Check sheet for the modelled part. Datum: model origin and axes. Units: mm. Face numbers are marked on the shaded views. Give positions to 0.01 mm unless a question says otherwise; leave off trailing zeros. Loops run counter-clockwise (first coordinate to the right, second up) from the corner with the lowest first, then second, coordinate; pieces in that order, holes last. Notation, with made-up numbers: (-34, 86.5) - (11, 86.5) arc R10 cw to (11, 97.5) - close; hole circle Ø7 at (67, 52). An arc over 180 degrees is marked (long way). Use CSV: the item, a comma, the result in double quotes.
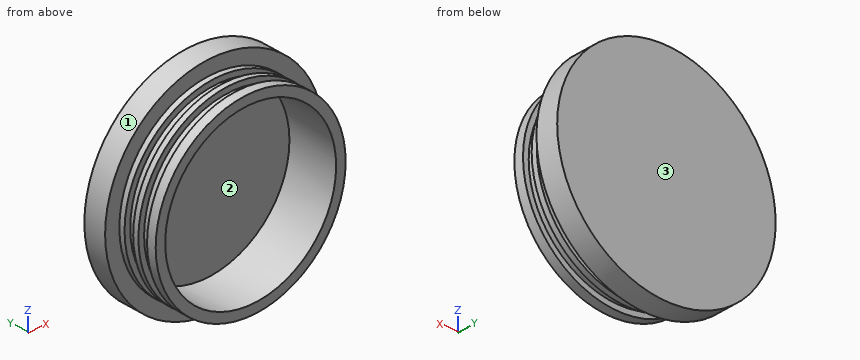
from build123d import *


with BuildPart() as part:
    # Esquisse1 → Révolution1 (revolve)
    with BuildSketch(Plane.XY):
        Polygon((0, 0), (45, 0), (45, -27), (50, -27), (50, -22), (47, -22), (47, -17), (50, -17), (50, -14), (47, -14), (47, -9), (50, -9), (50, -6), (57.5, -6), (57.5, 6), (0, 6), align=None)
    revolve(axis=Axis((0, 0, 0), (0, 1, 0)))


solid = part.part
1. Sectioned sample at B-B, the plane x = 0. Record the boundary of the cut face in (y, z).
Completed:
outline,"(-27, -50) - (-22, -50) - (-22, -47) - (-17, -47) - (-17, -50) - (-14, -50) - (-14, -47) - (-9, -47) - (-9, -50) - (-6, -50) - (-6, -57.5) - (6, -57.5) - (6, 57.5) - (-6, 57.5) - (-6, 50) - (-9, 50) - (-9, 47) - (-14, 47) - (-14, 50) - (-17, 50) - (-17, 47) - (-22, 47) - (-22, 50) - (-27, 50) - (-27, 45) - (0, 45) - (0, -45) - (-27, -45) - close"
2. Go/stop test with flat-tipped pins: pin 1 Ø6 at (y, z) = (-3.5, -10) entering from -X; pin 2 Ø1.5 at (y, z) = (-22, 45) entering from -X; pin 3 Ø5 at (y, z) = (-9.5, -36.5) entering from +X. Record where each tip stops, or that it passes through.
Completed:
pin 1,"stops at x = -57.07"
pin 2,"stops at x = -23.28"
pin 3,"stops at x = 36.61"
3. Sectioned sample at A-A, the plane z = 0. Record the boundary of the cut face in (x, y).
Completed:
outline,"(-57.5, -6) - (-50, -6) - (-50, -9) - (-47, -9) - (-47, -14) - (-50, -14) - (-50, -17) - (-47, -17) - (-47, -22) - (-50, -22) - (-50, -27) - (-45, -27) - (-45, 0) - (45, 0) - (45, -27) - (50, -27) - (50, -22) - (47, -22) - (47, -17) - (50, -17) - (50, -14) - (47, -14) - (47, -9) - (50, -9) - (50, -6) - (57.5, -6) - (57.5, 6) - (-57.5, 6) - close"
4. Release check for a two-part mould opening along Z. For the marked faces 1, 2 and 3 record: released by +Z, released by -Z, zero draft, split by the parting line, or undercut.
Completed:
face 1,"split by the parting line"
face 2,"undercut"
face 3,"zero draft"
5. Sectioned sample at C-C, the plane y = -1.5. Record the boundary of the cut face in (x, z), and give its area (3 significant figures).
Completed:
outline,"circle Ø115 at (0, 0); hole circle Ø90 at (0, 0)"
area,"4,030 mm²"
6. Scan lines: line 1 along Y through (x, z) = (-27.5, -41.5); line 2 along X through (y, z) = (-17.5, 0); line 3 along Z through (x, y) = (0, -8). Record each from-to range of solid material in increasing order.
Completed:
line 1,"y = -27 to -22, -17 to -14, -9 to 6"
line 2,"x = -47 to -45, 45 to 47"
line 3,"z = -50 to -45, 45 to 50"
7. Sectioned sample at D-D, the plane y = -10.5. Record the boundary of the cut face in (x, z), and give its area (3 significant figures).
Completed:
outline,"circle Ø94 at (0, 0); hole circle Ø90 at (0, 0)"
area,"578 mm²"
